```python
from build123d import *

# Parameters (mm, degrees)
SKETCH1_W                = 27.4
SKETCH1_H                = 45.4
SKETCH1_R                = 1.6
SKETCH1_R_2              = 1.599999998
BOSS_EXTRUDE1_DEPTH      = 5
BOSS_EXTRUDE1_DEPTH_BACK = 5.5


with BuildPart() as part:
    # Sketch1 → Boss-Extrude1 (new body, two sides)
    with BuildSketch(Plane.XY) as boss_extrude1_sk:
        with Locations((440.461848113, -60.80586409)):
            Rectangle(SKETCH1_W, SKETCH1_H)
        with Locations((430.461848113, -70.80586409)):
            Circle(SKETCH1_R, mode=Mode.SUBTRACT)
        with Locations((430.461848113, -50.80586409)):
            Circle(SKETCH1_R_2, mode=Mode.SUBTRACT)
        with Locations((450.461848113, -50.80586409)):
            Circle(SKETCH1_R_2, mode=Mode.SUBTRACT)
        with Locations((450.461848113, -70.80586409)):
            Circle(SKETCH1_R, mode=Mode.SUBTRACT)
    extrude(amount=BOSS_EXTRUDE1_DEPTH)
    extrude(boss_extrude1_sk.sketch, amount=-BOSS_EXTRUDE1_DEPTH_BACK)


solid = part.part
```
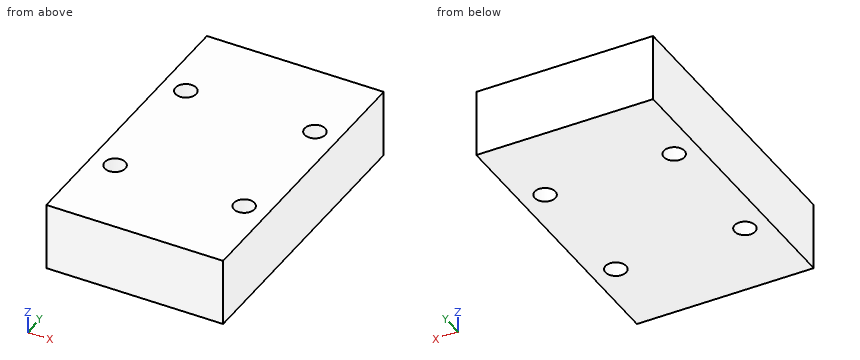
Geometry check sheet. Reference: the model listing, model coordinates, mm. Round coordinates to 2 decimals unless told otherwise and drop trailing zeros. Loops run counter-clockwise (first coordinate to the right, second up) from the corner with the lowest first, then second, coordinate; pieces in that order, holes last. Notation, with made-up numbers: (46.5, -19.75) - (100.5, -19.75) arc R27 ccw to (100.5, 10.25) - close; hole circle Ø2 at (31.25, 40.5). An arc over 180 degrees is marked (long way). Write item = value, one per line. Start each with the question number.
1. Section check A-A on y = -70. Enter the section's corners in (x, z), then the cut area to 3 significant figures.
2. Section check C-C on z = -2.5. Enter the section's corners in (x, y).
3. Section check B-B on x = 430.5. Enter the section's corners in (y, z).
4. Thickness scan on line 1 (Y direction, x = 429.5, z = -3.75); line 2 (Y direction, x = 450.75, z = -4.75); line 3 (X direction, y = -50, z = 0). Record the ranges inside material, lowest first.
Working result:
q1.outline = (426.76, -5.5) - (429.08, -5.5) - (429.08, 5) - (426.76, 5) - close; (431.84, -5.5) - (449.08, -5.5) - (449.08, 5) - (431.84, 5) - close; (451.84, -5.5) - (454.16, -5.5) - (454.16, 5) - (451.84, 5) - close
q1.area = 230 mm^2
q2.outline = (426.76, -83.51) - (454.16, -83.51) - (454.16, -38.11) - (426.76, -38.11) - close; hole circle Ø3.2 at (430.46, -70.81); hole circle Ø3.2 at (430.46, -50.81); hole circle Ø3.2 at (450.46, -70.81); hole circle Ø3.2 at (450.46, -50.81)
q3.outline = (-83.51, -5.5) - (-72.41, -5.5) - (-72.41, 5) - (-83.51, 5) - close; (-69.21, -5.5) - (-52.41, -5.5) - (-52.41, 5) - (-69.21, 5) - close; (-49.21, -5.5) - (-38.11, -5.5) - (-38.11, 5) - (-49.21, 5) - close
q4.line_1 = -83.51 to -72.08, -69.53 to -52.08, -49.53 to -38.11
q4.line_2 = -83.51 to -72.38, -69.23 to -52.38, -49.23 to -38.11
q4.line_3 = 426.76 to 429.08, 431.84 to 449.08, 451.84 to 454.16
